Verification items for the finished model (mm, model axes). A direction names the side the tool comes from. Give positions to 0.01 mm unless a question says otherwise; leave off trailing zeros. Answer in a Markdown table with one row per item. Add a question column.
Q1. Gauge pin test, flat ends, axial feed: P1, Ø10.5, axis at x = 8, y = -16, coming from the +Z side; P2, Ø11.5, axis at x = 2.5, z = 427, coming from the -Y side (3 decimals). Record the tip position at first contact, or that the pin passes through.
Q2. Set-up check for faces 1 (the face through (0, 0, 6)), 2 (the face through (0, -9.525, 427)): record each of +Z, -Z, +X, -X, +Y, -Y from which the full face is reachable in a straight line by a thin tool's end or side.
Q3. Material ranges on probe 1 along X at (y, z) = (-16.5, -65); probe 2 along Z at (x, y) = (-15, -10); probe 3 along X at (y, z) = (-17, -381), recorded low to high.
```python
from build123d import *

# Parameters (mm, degrees)
F0_W     = 38.1
F0_H     = 890.5875
F1_DEPTH = 19.05
F2_W     = 38.1
F2_H     = 38.1
F3_DEPTH = 9.525
F4_R     = 3.175


with BuildPart() as f1:
    # F0 (on Front) → F1 (new body)
    with BuildSketch(Plane.XZ):
        Rectangle(F0_W, F0_H)
    extrude(amount=F1_DEPTH)

    # F2 (on face) → F3 (cut)
    with BuildSketch(Plane.XZ.offset(19.05)):
        with Locations((0, 426.24375)):
            Rectangle(F2_W, F2_H)
    extrude(amount=-F3_DEPTH, mode=Mode.SUBTRACT)

    # F4
    f4_edges = [f1.edges().sort_by_distance(p)[0] for p in [
        (-19.05, -19.05, -19.05),
        (19.05, -19.05, -19.05),
    ]]
    fillet(f4_edges, radius=F4_R)


solid = f1.part
```
Taken from the geometry:
| question | item | result |
|---|---|---|
| 1 | P1 | stops at z = 407.19 |
| 1 | P2 | stops at y = -9.525 |
| 2 | face 1 | +Z, -Z, +X, -X, +Y |
| 2 | face 2 | +Z, +X, -X, -Y |
| 3 | probe 1 | x = -18.99 to 18.99 |
| 3 | probe 2 | z = -445.29 to 407.19 |
| 3 | probe 3 | x = -18.84 to 18.84 |
